Model file for the job. Use its own axes, mm. A direction names the side the tool comes from. Round coordinates to 2 decimals unless told otherwise and drop trailing zeros. Order: outer loops, then holes, each group sorted by start corner. A loop starts at its lowest first (then second) coordinate and runs counter-clockwise, first axis right, second up. Notation, with made-up numbers: (-14.75, -11) - (-1.75, -11) arc R18 cw to (-1.75, 22) - close; hole circle Ø9 at (-24, 27). An arc over 180 degrees is marked (long way). Write item = value, one per line.
```python
from build123d import *

# Parameters (mm, degrees)
SKETCH1_W                   = 152.4
SKETCH1_H                   = 50.8
BOSS_EXTRUDE1_DEPTH         = 6.604
CUT_EXTRUDE1_DEPTH          = 7.604
F_1_4_20_TAPPED_HOLE1_D     = 5.1054
F_1_4_20_TAPPED_HOLE1_DEPTH = 16.51
F_1_4_20_TAPPED_HOLE1_TIP   = 1.533816902
F_8_CLEARANCE_HOLE1_D       = 4.3053
F_8_CLEARANCE_HOLE1_DEPTH   = 7.62
F_8_CLEARANCE_HOLE1_TIP     = 1.293442612


with BuildPart() as part:
    # Sketch1 → Boss-Extrude1 (new body)
    with BuildSketch(Plane(origin=(0, 0, 0), x_dir=(1, 0, 0), z_dir=(0, 1, 0))):
        Rectangle(SKETCH1_W, SKETCH1_H)
    extrude(amount=BOSS_EXTRUDE1_DEPTH)

    # Sketch2 → Cut-Extrude1 (cut, through all)
    with BuildSketch(Plane(origin=(0, 6.604, 0), x_dir=(1, 0, 0), z_dir=(0, 1, 0))):
        with BuildLine():
            Line((-44.45, 25.4), (-31.75, 25.4))
            Line((-31.75, 25.4), (-31.75, 15.875))
            ThreePointArc((-31.75, 15.875), (-32.67993597, 13.62993597), (-34.925, 12.7))
            Line((-34.925, 12.7), (-41.275, 12.7))
            ThreePointArc((-41.275, 12.7), (-43.52006403, 13.62993597), (-44.45, 15.875))
            Line((-44.45, 15.875), (-44.45, 25.4))
        make_face()
    cut_extrude1 = extrude(amount=-CUT_EXTRUDE1_DEPTH, mode=Mode.SUBTRACT)

    # Mirror1: Cut-Extrude1 across plane
    add(cut_extrude1.mirror(Plane(origin=(0, 0, 0), x_dir=(0, 0, 1), z_dir=(1, 0, 0))), mode=Mode.SUBTRACT)

    # 1/4-20 Tapped Hole1
    with Locations(Plane(origin=(0, 6.604, 0), x_dir=(1, 0, 0), z_dir=(0, 1, 0))):
        with Locations((-60.325, 0), (60.325, 0)):
            Hole(F_1_4_20_TAPPED_HOLE1_D / 2, depth=F_1_4_20_TAPPED_HOLE1_DEPTH)
            with Locations((0, 0, -(F_1_4_20_TAPPED_HOLE1_DEPTH + F_1_4_20_TAPPED_HOLE1_TIP / 2))):  # 118° drill point
                Cone(0, F_1_4_20_TAPPED_HOLE1_D / 2, F_1_4_20_TAPPED_HOLE1_TIP, mode=Mode.SUBTRACT)

    # #8 Clearance Hole1
    with Locations(Plane(origin=(0, 6.604, 0), x_dir=(1, 0, 0), z_dir=(0, 1, 0))):
        with Locations((-19.05, 12.7), (-19.05, -12.7), (19.05, 12.7), (19.05, -12.7)):
            Hole(F_8_CLEARANCE_HOLE1_D / 2, depth=F_8_CLEARANCE_HOLE1_DEPTH)
            with Locations((0, 0, -(F_8_CLEARANCE_HOLE1_DEPTH + F_8_CLEARANCE_HOLE1_TIP / 2))):  # 118° drill point
                Cone(0, F_8_CLEARANCE_HOLE1_D / 2, F_8_CLEARANCE_HOLE1_TIP, mode=Mode.SUBTRACT)


solid = part.part
```
1) Cut at A-A (x = -19.05). Write the cut outline in (y, z), and give its area (3 significant figures).
Conclusion:
outline = (0, -25.4) - (6.6, -25.4) - (6.6, -14.85) - (0, -14.85) - close; (0, -10.55) - (6.6, -10.55) - (6.6, 10.55) - (0, 10.55) - close; (0, 14.85) - (6.6, 14.85) - (6.6, 25.4) - (0, 25.4) - close
area = 279 mm^2
2) 3-axis set-ups, long thin cutter, end or side, ignore diameter. For faces 1 (the face through (-1, 6.604, 0)), 2 (the face through (38, 3, -12.7)): which of +Z, -Z, +X, -X, +Y, -Y reach the whole face in a straight line?
Conclusion:
face_1 = +Z, -Z, +X, -X, +Y
face_2 = -Z, +Y, -Y
3) Cut at B-B (z = 0). Write the cut outline in (x, y), and give its area (3 significant figures).
Conclusion:
outline = (-76.2, 0) - (-62.88, 0) - (-62.88, 6.6) - (-76.2, 6.6) - close; (-57.77, 0) - (57.77, 0) - (57.77, 6.6) - (-57.77, 6.6) - close; (62.88, 0) - (76.2, 0) - (76.2, 6.6) - (62.88, 6.6) - close
area = 939 mm^2
4) Mould opens along X. For faces 3 (the face through (62.875, 3.256, -0.112)), 4 (the face through (76.2, 3, 0)), 5 (the face through (-1, 0, 0)) say: +X half, -X half, draft (parallel to the pull), parting line (faces both ways), or undercut.
Conclusion:
face_3 = undercut
face_4 = +X half
face_5 = draft
5) Cut at C-C (y = 3.75). Write the cut outline in (x, z) (3 decimals), and give its area (3 significant figures).
Conclusion:
outline = (-76.2, -25.4) - (-44.45, -25.4) - (-44.45, -15.875) arc R3.175 cw to (-41.275, -12.7) - (-34.925, -12.7) arc R3.175 cw to (-31.75, -15.875) - (-31.75, -25.4) - (31.75, -25.4) - (31.75, -15.875) arc R3.175 cw to (34.925, -12.7) - (41.275, -12.7) arc R3.175 cw to (44.45, -15.875) - (44.45, -25.4) - (76.2, -25.4) - (76.2, 25.4) - (-76.2, 25.4) - close; hole circle Ø5.105 at (-60.325, 0); hole circle Ø4.305 at (-19.05, -12.7); hole circle Ø4.305 at (-19.05, 12.7); hole circle Ø4.305 at (19.05, -12.7); hole circle Ø4.305 at (19.05, 12.7); hole circle Ø5.105 at (60.325, 0)
area = 7,330 mm^2
6) Flat gauge pin, fed straight in: pin 1 Ø1.9 at (x, y) = (37, 4.5) entering from -Z. Where does the tip first touch, or does it go through?
Conclusion:
pin_1 = -12.7
7) Wall check: line 1 along Z through (x, y) = (19.05, 2.75); line 2 along X through (y, z) = (3.25, 12.7); line 3 along X through (y, z) = (3.5, -23). Give the ranges that are in metal, low to high.
Conclusion:
line_1 = -25.4 to -14.85, -10.55 to 10.55, 14.85 to 25.4
line_2 = -76.2 to -21.2, -16.9 to 16.9, 21.2 to 76.2
line_3 = -76.2 to -44.45, -31.75 to 31.75, 44.45 to 76.2
